Can you work these out from the model? Positions are in its coordinate system, mm. Face numbers are marked on the shaded views. A direction names the side the tool comes from. Give positions to 0.01 mm unless a question says otherwise; leave off trailing zeros. Order: outer loops, then holes, each group sorted by start corner. A loop starts at its lowest first (then second) coordinate and runs counter-clockwise, first axis right, second up. Notation, with made-up numbers: M 35.5,18 L 75.5,18 A15 cw 75.5,36 Z; hole C 47.5,-40 d3. An arc over 180 degrees is marked long. Answer as a JSON object with one key per item and string values.
```python
from build123d import *

# Parameters (mm, degrees)
F0_W     = 4
F0_H     = 38.3
F0_R     = 1.75
F0_R_2   = 11.25
F1_DEPTH = 4
F3_DEPTH = 20
F4_R     = 2.75
F5_DEPTH = 4
F6_R     = 2.5


with BuildPart() as f1:
    # F0 (on Top) → F1 (new body)
    with BuildSketch(Plane.XY):
        with Locations((-23.15, 2)):
            Rectangle(F0_W, F0_H)
        Polygon((21.15, 21.15), (-21.15, 21.15), (-21.15, -17.15), (-21.15, -21.15), (21.15, -21.15), (21.15, -17.15), align=None)
        with Locations((-15.495, -15.495)):
            Circle(F0_R, mode=Mode.SUBTRACT)
        with Locations((15.495, -15.495)):
            Circle(F0_R, mode=Mode.SUBTRACT)
        with Locations((-15.495, 15.495)):
            Circle(F0_R, mode=Mode.SUBTRACT)
        Circle(F0_R_2, mode=Mode.SUBTRACT)
        with Locations((15.495, 15.495)):
            Circle(F0_R, mode=Mode.SUBTRACT)
        with Locations((23.15, 2)):
            Rectangle(F0_W, F0_H)
        Polygon((-21.15, -21.15), (-21.15, -17.15), (-25.15, -17.15), (-40.15, -17.15), (-40.15, -21.15), align=None)
        Polygon((25.15, -17.15), (21.15, -17.15), (21.15, -21.15), (40.15, -21.15), (40.15, -17.15), align=None)
    extrude(amount=F1_DEPTH)

    # F2 (on face) → F3 (join)
    with BuildSketch(Plane(origin=(0, 0, 0), x_dir=(1, 0, 0), z_dir=(0, 0, -1))):
        Polygon((-25.15, -21.15), (-21.15, -21.15), (-21.15, 17.15), (-21.15, 21.15), (-40.15, 21.15), (-40.15, 17.15), (-25.15, 17.15), align=None)
        Polygon((21.15, 17.15), (21.15, -21.15), (25.15, -21.15), (25.15, 17.15), (40.15, 17.15), (40.15, 21.15), (21.15, 21.15), align=None)
    extrude(amount=F3_DEPTH)

    # F4 (on face) → F5 (cut, through all)
    with BuildSketch(Plane.XZ.offset(21.15)):
        with Locations((-32.65, -10)):
            Circle(F4_R)
        with Locations((32.65, -10)):
            Circle(F4_R)
    extrude(amount=-F5_DEPTH, mode=Mode.SUBTRACT)

    # F6
    f6_edges = [f1.edges().sort_by_distance(p)[0] for p in [
        (-40.15, -19.15, 4),
        (-40.15, -19.15, -20),
        (40.15, -19.15, -20),
        (40.15, -19.15, 4),
        (25.15, -17.15, -8),
        (-25.15, -17.15, -8),
        (21.15, -21.15, -10),
        (-21.15, -21.15, -10),
    ]]
    fillet(f6_edges, radius=F6_R)


solid = f1.part
```
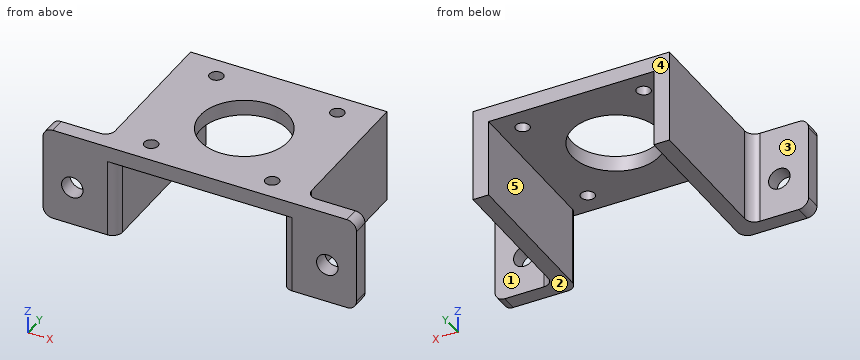
1) I want a section at A-A on x = 0. Write out the boundary of the cut face in (y, z), and give its area (3 significant figures).
Results found:
{"outline": "M -21.15,0 L -11.25,0 L -11.25,4 L -21.15,4 Z; M 11.25,0 L 21.15,0 L 21.15,4 L 11.25,4 Z", "area": "79.2 mm²"}
2) I need wall thicknesses on L1, parallel to X at y = -3, z = -7.5; L2, parallel to Y at x = -34, z = -14; L3, parallel to X at y = -18, z = -1. Which ranges of each line are inside material? Lowest first, please.
Results found:
{"L1": "x = -25.15 to -21.15, 21.15 to 25.15", "L2": "y = -21.15 to -17.15", "L3": "x = -40.15 to -21.15, 21.15 to 40.15"}
3) I want a section at D-D on z = -15.5. Write out the boundary of the cut face in (x, y).
Results found:
{"outline": "M -40.15,-21.15 L -23.65,-21.15 A2.5 ccw -21.15,-18.65 L -21.15,21.15 L -25.15,21.15 L -25.15,-14.65 A2.5 cw -27.65,-17.15 L -40.15,-17.15 Z; M 21.15,-18.65 A2.5 ccw 23.65,-21.15 L 40.15,-21.15 L 40.15,-17.15 L 27.65,-17.15 A2.5 cw 25.15,-14.65 L 25.15,21.15 L 21.15,21.15 Z"}
4) For the marked faces 1, 2, 3, 4 and 5, which set-ups out of +Z, -Z, +X, -X, +Y, -Y let a thin tool reach every point of the face, with its end or its side?
Results found:
{"face 1": "+Z, -Z, +X, +Y", "face 2": "-Z, +X, -X, +Y, -Y", "face 3": "+Z, -Z, -X, +Y", "face 4": "+Z, -Z, +X, -X, +Y", "face 5": "-Z, +Y, -Y"}
5) I want a section at C-C on y = 0. Write out the boundary of the cut face in (x, z), and give its area (3 significant figures).
Results found:
{"outline": "M -25.15,-20 L -21.15,-20 L -21.15,0 L -11.25,0 L -11.25,4 L -25.15,4 Z; M 11.25,0 L 21.15,0 L 21.15,-20 L 25.15,-20 L 25.15,4 L 11.25,4 Z", "area": "271 mm²"}
6) I want a section at B-B on z = -10. Write out the boundary of the cut face in (x, y), and give its area (3 significant figures).
Results found:
{"outline": "M -40.15,-21.15 L -35.4,-21.15 L -35.4,-17.15 L -40.15,-17.15 Z; M -29.9,-21.15 L -23.65,-21.15 A2.5 ccw -21.15,-18.65 L -21.15,21.15 L -25.15,21.15 L -25.15,-14.65 A2.5 cw -27.65,-17.15 L -29.9,-17.15 Z; M 21.15,-18.65 A2.5 ccw 23.65,-21.15 L 29.9,-21.15 L 29.9,-17.15 L 27.65,-17.15 A2.5 cw 25.15,-14.65 L 25.15,21.15 L 21.15,21.15 Z; M 35.4,-21.15 L 40.15,-21.15 L 40.15,-17.15 L 35.4,-17.15 Z", "area": "414 mm²"}
7) I'm going to push flat-ended pins straight in: pin 1 Ø7 at (x, z) = (-32.65, -10) entering from -Y; pin 2 Ø5 at (y, z) = (-4, -16) entering from +X; pin 3 Ø2 at (x, y) = (-15.495, 15.495) entering from -Z; pin 4 Ø3 at (y, z) = (-13, -6) entering from -X. Where does each tip first touch, or does it pass through?
Results found:
{"pin 1": "stops at y = -21.15", "pin 2": "stops at x = 25.15", "pin 3": "passes through", "pin 4": "stops at x = -25.15"}
